Here's the drawing with two shaded views (mm, measured from the low corner). I have some questions. A direction names the side the tool comes from. Coordinates: 2 decimals unless noted, no trailing zeros. Write each loop counter-clockwise with the first axis right and the second up, starting at its lowest first coordinate (ties: lowest second). Pieces come first, ordered by that corner, then holes.
Item 1: If we section it at A-A (y = 12.5): Please give me the cut outline in (x, z).
Item 2: For the marked faces 1 and 2, which set-ups out of +Z, -Z, +X, -X, +Y, -Y let a thin tool reach every point of the face, with its end or its side?
Item 3: I'm going to push flat-ended pins straight in: pin 1 Ø6 at (x, z) = (35, 22) entering from +Y; pin 2 Ø12 at (x, y) = (51.5, 18) entering from +Z. Where does each tip first touch, or does it pass through?
Item 4: If I drill on line 1 (Z direction, x = 9, y = 66); line 2 (Y direction, x = 3, z = 9); line 3 (Z direction, x = 40, y = 62), over which ranges is the centre line in solid material (lowest first)?
Item 5: If we section it at D-D (z = 59): Please give me the cut outline in (x, y), then the cut area to 3 significant figures.
Item 6: If we section it at C-C (x = 9): Count the separate pieces of the cut face and the enclosed holes in it, then the cut area to 3 significant figures.
Item 7: If we section it at B-B (z = 35.5): Please give me the cut outline in (x, y).
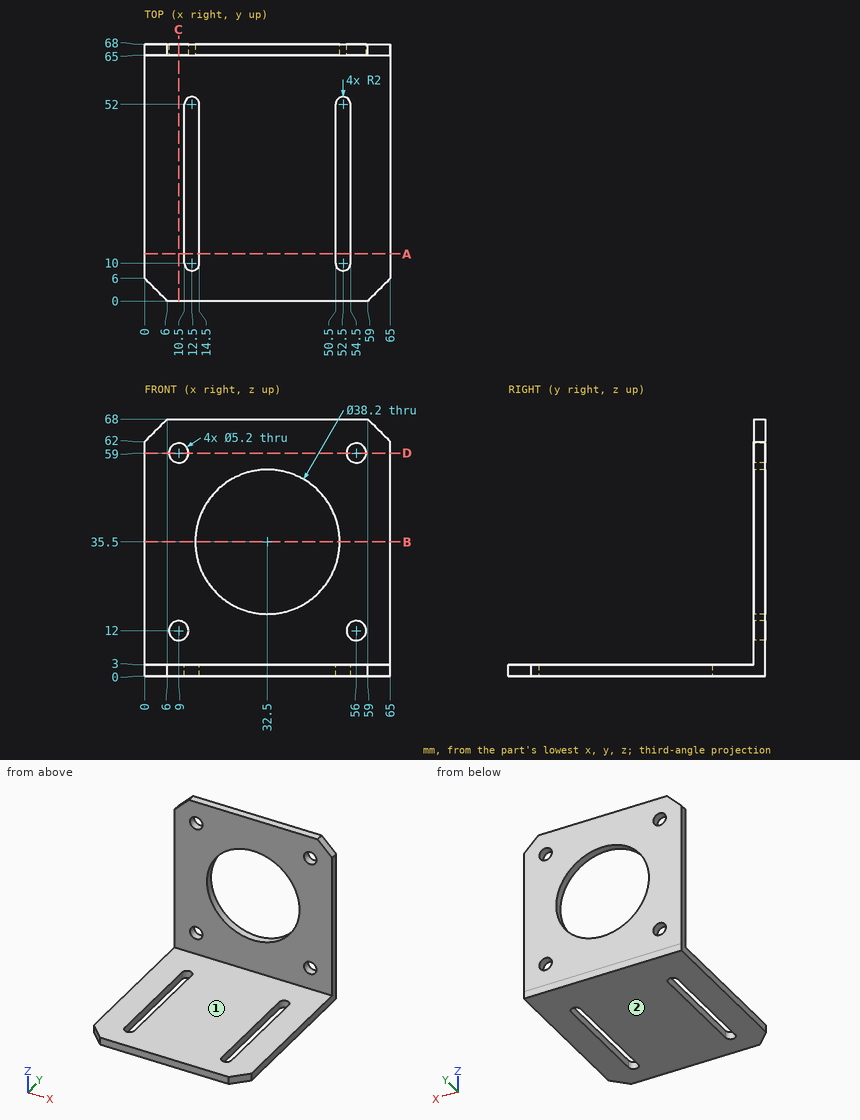
Answer list:
1. outline: (0, 0) - (10.5, 0) - (10.5, 3) - (0, 3) - close; (14.5, 0) - (50.5, 0) - (50.5, 3) - (14.5, 3) - close; (54.5, 0) - (65, 0) - (65, 3) - (54.5, 3) - close
2. face 1: +Z, +X, -X, -Y
2. face 2: -Z, +X, -X, +Y, -Y
3. pin 1: passes through
3. pin 2: stops at z = 3
4. line 1: z = 0 to 9.4, 14.6 to 56.4, 61.6 to 68
4. line 2: y = 65 to 68
4. line 3: z = 0 to 3
5. outline: (0, 65) - (6.4, 65) - (6.4, 68) - (0, 68) - close; (11.6, 65) - (53.4, 65) - (53.4, 68) - (11.6, 68) - close; (58.6, 65) - (65, 65) - (65, 68) - (58.6, 68) - close
5. area: 164 mm2
6. separate pieces: 3
6. enclosed holes: 0
6. area: 368 mm2
7. outline: (0, 65) - (13.4, 65) - (13.4, 68) - (0, 68) - close; (51.6, 65) - (65, 65) - (65, 68) - (51.6, 68) - close
